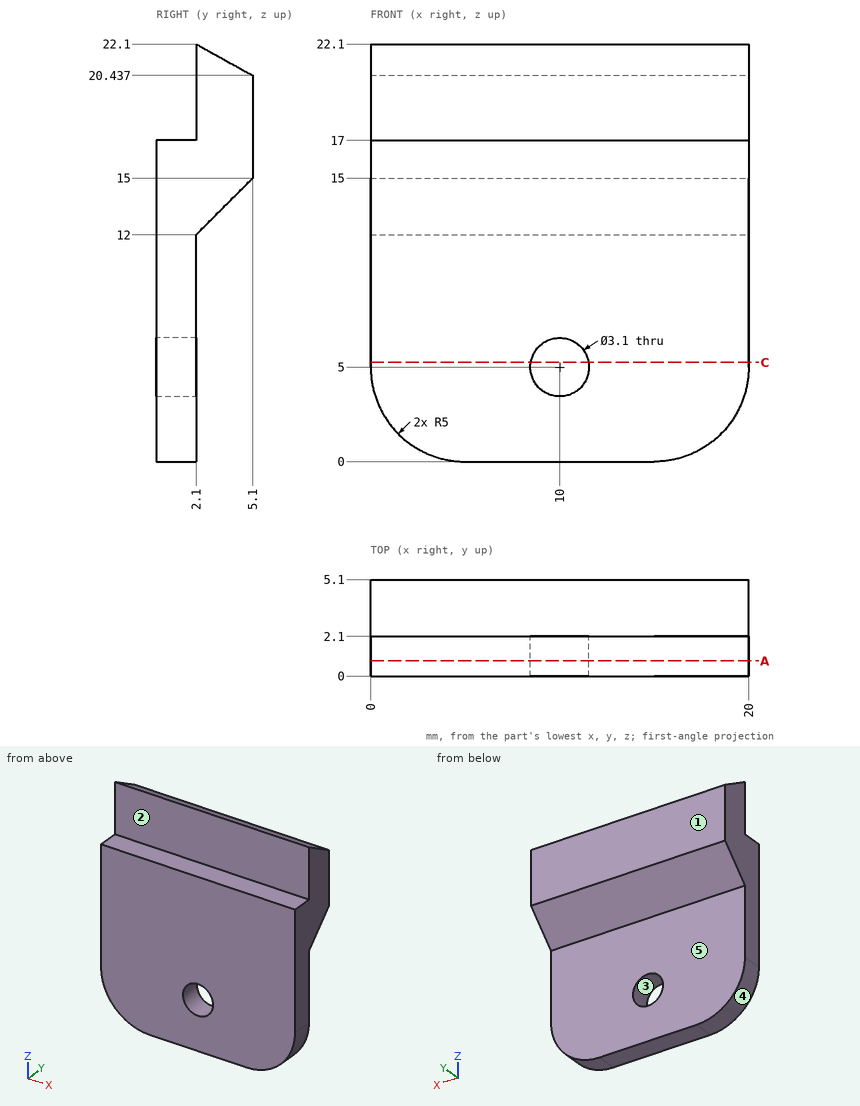
Verification items for this drawing (mm, ordinates from the low corner). A direction names the side the tool comes from. Give positions to 0.01 mm unless a question says otherwise; leave off trailing zeros. Order: outer loops, then holes, each group sorted by start corner. A loop starts at its lowest first (then second) coordinate and runs counter-clockwise, first axis right, second up.
1) Cross-section at A-A (y = 0.8). Record the boundary of the cut face in (x, z), then the cut area to 3 significant figures.
Results are:
outline: (0, 5) arc R5 ccw to (5, 0) - (15, 0) arc R5 ccw to (20, 5) - (20, 17) - (0, 17) - close; hole circle Ø3.1 at (10, 5)
area: 322 mm2
2) Tool access check on the marked faces 1 and 2. Record the directions out of +Z, -Z, +X, -X, +Y, -Y that give a thin tool (end or side, any length) a straight path to the whole face; none if there is none.
Results are:
face 1: +Z, -Z, +X, -X, +Y
face 2: +Z, +X, -X, -Y
3) Material ranges on probe 1 along X at (y, z) = (1.1, 5); probe 2 along Z at (x, y) = (13.25, 0.55); probe 3 along Y at (x, z) = (12, 9.25), recorded low to high.
Results are:
probe 1: x = 0 to 8.45, 11.55 to 20
probe 2: z = 0 to 17
probe 3: y = 0 to 2.1
4) Draft check along Z on the marked faces 3, 4 and 5. Enter one of: released by +Z, released by -Z, zero draft, split by the parting line, or undercut.
Results are:
face 3: undercut
face 4: released by -Z
face 5: zero draft
5) Gauge pin test, flat ends, axial feed: pin 1 (3 mm diameter, centred on x = 15.5, y = 1.5, fed in from -Z); pin 2 (1.7 mm diameter, centred on x = 7.5, y = 1.5, fed in from +Z); pin 3 (5 mm diameter, centred on x = 10.5, z = 11, fed in from +Y); pin 4 (1.5 mm diameter, centred on x = 14.5, z = 20, fed in from -Y). Record the tip position at first contact, or that the pin passes through.
Results are:
pin 1: stops at z = 0
pin 2: stops at z = 22.1
pin 3: stops at y = 3.6
pin 4: stops at y = 2.1
6) Cross-section at C-C (z = 5.25). Record the boundary of the cut face in (x, y), then the cut area to 3 significant figures.
Results are:
outline: (0, 0) - (8.47, 0) - (8.47, 2.1) - (0, 2.1) - close; (11.53, 0) - (20, 0) - (20, 2.1) - (11.53, 2.1) - close
area: 35.6 mm2
